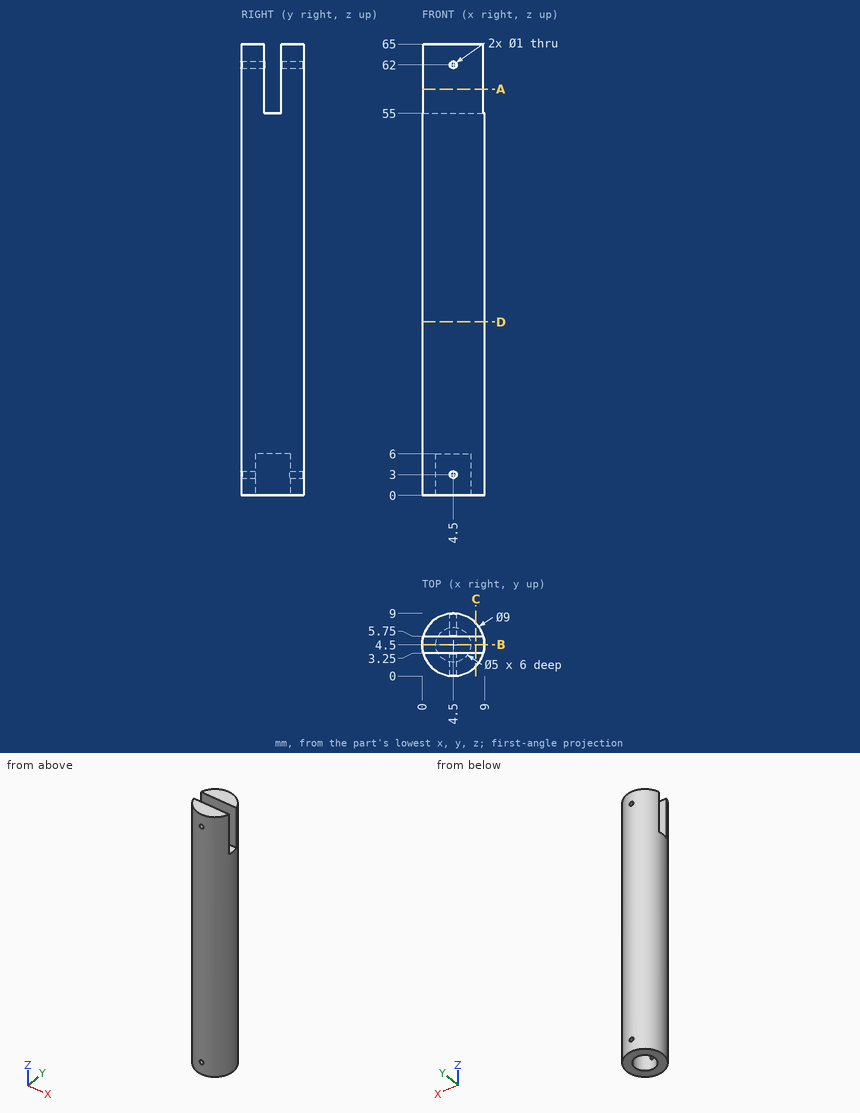
The figure shows three views and two pictorial views of one solid part (mm, origin at its lowest corner). Answer the questions. Round coordinates to 2 decimals unless told otherwise and drop trailing zeros. Write each loop counter-clockwise with the first axis right and the second up, starting at its lowest first coordinate (ties: lowest second). Pieces come first, ordered by that corner, then holes. Notation, with made-up numbers: (73.5, 41.25) -> (113.5, 41.25) arc R22 cw to (113.5, 57.25) -> close; hole circle Ø11 at (55, -8). An arc over 180 degrees is marked (long way). Answer as a JSON object with one key per item and string values. Group by question number.
Q1. Section C-C (x = 7.75) is taken. Write down the section's boundary in (y, z).
Q2. Section B-B (y = 4.5) is taken. Write down the section's boundary in (x, z), plus the area to 3 significant figures.
Q3. Section D-D (z = 25) is taken. Write down the section's boundary in (x, y).
Q4. Section A-A (z = 58.5) is taken. Write down the section's boundary in (x, y).
Q5. Each of these flat-tipped pins is pushed along its axis until it touches: pin 1 Ø1.3 at (x, y) = (6, 4.5) entering from +Z; pin 2 Ø5 at (x, z) = (6, 56) entering from -Y; pin 3 Ø4 at (x, y) = (4.5, 4.5) entering from -Z; pin 4 Ø1.5 at (x, z) = (5.5, 52) entering from +Y. Where does it stop, or does it pass through?
Q6. Straight lines are drawn through the part: line 1 along Y through (x, z) = (8.25, 39); line 2 along Z through (x, y) = (3.75, 6.5); line 3 along X through (y, z) = (2.55, 62). For each, find the intervals that lie inside material, in ascending order.
Check values:
{
 "1": {"outline": "(1.39, 0) -> (7.61, 0) -> (7.61, 65) -> (5.75, 65) -> (5.75, 55) -> (3.25, 55) -> (3.25, 65) -> (1.39, 65) -> close"},
 "2": {"outline": "(0, 0) -> (2, 0) -> (2, 6) -> (7, 6) -> (7, 0) -> (9, 0) -> (9, 55) -> (0, 55) -> close", "area": "465 mm^2"},
 "3": {"outline": "circle Ø9 at (4.5, 4.5)"},
 "4": {"outline": "(0.18, 3.25) arc R4.5 ccw to (8.82, 3.25) -> close; (0.18, 5.75) -> (8.82, 5.75) arc R4.5 ccw to start"},
 "5": {"pin 1": "z = 55", "pin 2": "y = 0", "pin 3": "z = 6", "pin 4": "y = 8.99"},
 "6": {"line 1": "2.01 to 6.99", "line 2": "6 to 65", "line 3": "0.44 to 4, 5 to 8.56"}
}
